from build123d import *

# Parameters (mm, degrees)
SKETCH_1_R       = 25
SKETCH_1_R_2     = 2.05
EXTRUDE_1_DEPTH  = 5
SKETCH_2_R       = 10
EXTRUDE_2_DEPTH  = 60
FILLET_1_R       = 2
SKETCH_4_R       = 14
EXTRUDE_3_DEPTH  = 15
CHAMFER_1_SIZE   = 15
CHAMFER_1_SIZE_2 = 4


with BuildPart() as part:
    # 草图1 → 凸台-拉伸1 (new body)
    with BuildSketch(Plane.XY):
        Circle(SKETCH_1_R)
        with Locations((0, 21.75)):
            Circle(SKETCH_1_R_2, mode=Mode.SUBTRACT)
        with Locations((16.661466638, 13.980630511)):
            Circle(SKETCH_1_R_2, mode=Mode.SUBTRACT)
        with Locations((-16.661466638, 13.980630511)):
            Circle(SKETCH_1_R_2, mode=Mode.SUBTRACT)
        with Locations(Location((16.661466638, -13.980630511, 0), (0, 0, 180))):
            Circle(SKETCH_1_R_2, mode=Mode.SUBTRACT)
        with Locations(Location((0, -21.75, 0), (0, 0, 180))):
            Circle(SKETCH_1_R_2, mode=Mode.SUBTRACT)
        with Locations(Location((-16.661466638, -13.980630511, 0), (0, 0, 180))):
            Circle(SKETCH_1_R_2, mode=Mode.SUBTRACT)
        with Locations((8.625, 14.938938215)):
            Circle(SKETCH_1_R_2, mode=Mode.SUBTRACT)
        with Locations((17.25, 0)):
            Circle(SKETCH_1_R_2, mode=Mode.SUBTRACT)
        with Locations((8.625, -14.938938215)):
            Circle(SKETCH_1_R_2, mode=Mode.SUBTRACT)
        with Locations((-8.625, -14.938938215)):
            Circle(SKETCH_1_R_2, mode=Mode.SUBTRACT)
        with Locations((-17.25, 0)):
            Circle(SKETCH_1_R_2, mode=Mode.SUBTRACT)
        with Locations((-8.625, 14.938938215)):
            Circle(SKETCH_1_R_2, mode=Mode.SUBTRACT)
    extrude(amount=EXTRUDE_1_DEPTH)

    # 草图2 → 凸台-拉伸2 (add)
    with BuildSketch(Plane.XY.offset(5)):
        with Locations(Location((0, 0, 0), (0, 0, 180))):
            Circle(SKETCH_2_R)
    extrude(amount=EXTRUDE_2_DEPTH)

    # 圆角1
    fillet_1_edges = [part.edges().sort_by_distance(p)[0] for p in [
        (10, 0, 5),
    ]]
    fillet(fillet_1_edges, radius=FILLET_1_R)

    # 草图4 → 凸台-拉伸3 (add)
    with BuildSketch(Plane.XY.offset(65)):
        Circle(SKETCH_4_R)
    extrude(amount=-EXTRUDE_3_DEPTH)

    # 倒角1
    # the kernel refuses this chamfer: 15, 4 mm, written as the material it adds along each edge
    with BuildSketch(Plane(origin=(0, 0, 50), x_dir=(-1, 0, 0), z_dir=(0, -1, 0))) as chamfer_1_piece_1_section:
        Polygon((10, CHAMFER_1_SIZE), (10 + CHAMFER_1_SIZE_2, 0), (10, 0), align=None)
    chamfer_1_piece_1 = revolve(axis=Axis((0, 0, 50), (0, 0, -1)), mode=Mode.PRIVATE)
    chamfer_1_piece_1 = chamfer_1_piece_1 & Plane(origin=(0, 0, 42.245414998), x_dir=(1, 0, 0), z_dir=(0, 0, 1)) * Cylinder(14, 60, mode=Mode.PRIVATE)
    add(chamfer_1_piece_1)


solid = part.part
Source: CAD feature listing. Evaluate the final solid. Frame: model axes, mm. A direction names the side the tool comes from. Give positions to 0.01 mm unless a question says otherwise; leave off trailing zeros. Write each loop counter-clockwise with the first axis right and the second up, starting at its lowest first coordinate (ties: lowest second). Pieces come first, ordered by that corner, then holes. Notation, with made-up numbers: (34, -28) - (61, -28) arc R17 ccw to (61, -13) - close; hole circle Ø7 at (29, 9.5). An arc over 180 degrees is marked (long way). Write item = value, one per line. Start each with the question number.
Q1. Reachability of faces 4 (the cylindrical face through (14.706, -14.596, 2.465)), 5 (the cylindrical face through (12.932, -5.362, 57.605)), 6 (the flat face through (-6, -11, 5)) from +Z, -Z, +X, -X, +Y, -Y: full face, straight path, thin tool, end or side. Return the list, or none.
Q2. Cut plane D-D, the plane y = 21.75. Return loops of the section in (x, z), then the cut area to 3 significant figures.
Q3. Cut plane A-A, the plane x = 0. Return loops of the section in (y, z), then the cut area to 3 significant figures.
Q4. Cut plane B-B, the plane y = 0. Return loops of the section in (x, z).
Q5. Pin query (flat end, axial travel): pin 1 Ø4.5 at (x, y) = (0, 21.75) entering from +Z; pin 2 Ø1 at (y, z) = (-6, 41) entering from +X; pin 3 Ø3.5 at (x, y) = (-16.66, -13.98) entering from -Z; pin 4 Ø12 at (y, z) = (4, 28.5) entering from -X. Return the tip coordinate at first contact, or that it passes through.
Q6. Cut plane C-C, the plane x = -17.25. Return loops of the section in (y, z).
Q7. Draft query along Z for faces 1 (the conical face through (8.21, 7.53, 39.27)), 2 (the cylindrical face through (18.617, 14.596, 2.465)), 3 (the flat face through (0, 0, 65)). Return one class per face: +Z half, -Z half, draft (parallel to the pull), parting line (faces both ways), or undercut.
Q8. Material intervals for probe 1 along Z at (x, y) = (11, -11.5); probe 2 along Y at (x, z) = (5.5, 52.5); probe 3 along Y at (x, z) = (6, 25), sorted ascending.
Computed values:
q1.face_4 = +Z, -Z
q1.face_5 = +Z
q1.face_6 = none
q2.outline = (-12.33, 0) - (-2.05, 0) - (-2.05, 5) - (-12.33, 5) - close; (2.05, 0) - (12.33, 0) - (12.33, 5) - (2.05, 5) - close
q2.area = 103 mm²
q3.outline = (-25, 0) - (-23.8, 0) - (-23.8, 5) - (-25, 5) - close; (-19.7, 0) - (19.7, 0) - (19.7, 5) - (12, 5) arc R2 cw to (10, 7) - (10, 35) - (14, 50) - (14, 65) - (-14, 65) - (-14, 50) - (-10, 35) - (-10, 7) arc R2 cw to (-12, 5) - (-19.7, 5) - close; (23.8, 0) - (25, 0) - (25, 5) - (23.8, 5) - close
q3.area = 1,590 mm²
q4.outline = (-25, 0) - (-19.3, 0) - (-19.3, 5) - (-25, 5) - close; (-15.2, 0) - (15.2, 0) - (15.2, 5) - (12, 5) arc R2 cw to (10, 7) - (10, 35) - (14, 50) - (14, 65) - (-14, 65) - (-14, 50) - (-10, 35) - (-10, 7) arc R2 cw to (-12, 5) - (-15.2, 5) - close; (19.3, 0) - (25, 0) - (25, 5) - (19.3, 5) - close
q5.pin_1 = 5
q5.pin_2 = 10.25
q5.pin_3 = through
q5.pin_4 = -10
q6.outline = (-18.1, 0) - (-15.94, 0) - (-15.94, 5) - (-18.1, 5) - close; (-12.02, 0) - (-2.05, 0) - (-2.05, 5) - (-12.02, 5) - close; (2.05, 0) - (12.02, 0) - (12.02, 5) - (2.05, 5) - close; (15.94, 0) - (18.1, 0) - (18.1, 5) - (15.94, 5) - close
q7.face_1 = undercut
q7.face_2 = draft
q7.face_3 = +Z half
q8.probe_1 = 0 to 5
q8.probe_2 = -12.87 to 12.87
q8.probe_3 = -8 to 8
